Design review of the part built by this model. Coordinates are the model's own, in mm. A direction names the side the tool comes from. Coordinates: 2 decimals unless noted, no trailing zeros. Order: outer loops, then holes, each group sorted by start corner. A loop starts at its lowest first (then second) coordinate and runs counter-clockwise, first axis right, second up. Notation, with made-up numbers: (-8.75, 62.25) -> (1.25, 62.25) arc R19 ccw to (1.25, 82.25) -> close; hole circle Ø3 at (61, -38.75). An arc over 180 degrees is marked (long way). Use a Markdown table: item, result. Add a question column.
Q1. Machinability: for faces 4 (the face through (-3.4, 12.3, 7.5)), 5 (the face through (2.17, -9.76, -4.89)), 6 (the face through (-11.923, 3.755, -7.423)), which of the approach directions +Z, -Z, +X, -X, +Y, -Y give a long, thin tool a straight path to every point of the face, cutting with its end or side? Answer none if there is none.
Q2. Add section A-A (x = 0). State the section outline as (y, z) points.
Q3. Add section D-D (z = 3.75). State the section outline as (x, y) points.
Q4. Insertion check: pin 1 (2 mm diameter, centred on y = 10.5, z = 5, fed in from -X); pin 2 (4 mm diameter, centred on x = -6, z = 3.5, fed in from +Y); pin 3 (1 mm diameter, centred on x = 2.5, z = 0, fed in from -Y). Each pin has a flat end and moves straight along its axis. Give the tip position at first contact, or say it passes through.
Q5. The part is to be moulded in two halves that separate along Y. For faces 1 (the face through (-14.985, 0.66, 3.698)), 2 (the face through (0, 0, -15)), 3 (the face through (11.923, 3.755, 4.965)), say which applies: pulls with the +Y half, pulls with the -Y half, needs draft (parallel to the pull), parting line crosses it, or undercut.
Q6. Add section C-C (z = -3). State the section outline as (x, y) points.
Q7. Wall thickness on probe 1 along Y at (x, z) = (0, 5.65); probe 2 along Z at (x, y) = (-6, -5.5); probe 3 along X at (y, z) = (8, 0.5): over which ranges is each line inside the solid? List them lowest first.
from build123d import *

# Parameters (mm, degrees)
ESBO_O1_R                = 15
RESSALTO_EXTRUS_O1_DEPTH = 7.5
ESBO_O2_R                = 12.5
RESSALTO_EXTRUS_O2_DEPTH = 15
CASCA1_T                 = -2.5
FILETE2_R                = 2


with BuildPart() as part:
    # Esboço1 → Ressalto-extrusão1 (new body)
    with BuildSketch(Plane.XY):
        Circle(ESBO_O1_R)
    extrude(amount=RESSALTO_EXTRUS_O1_DEPTH)

    # Esboço2 → Ressalto-extrusão2 (add)
    with BuildSketch(Plane(origin=(0, 0, 0), x_dir=(-1, 0, 0), z_dir=(0, 0, -1))):
        Circle(ESBO_O2_R)
    extrude(amount=RESSALTO_EXTRUS_O2_DEPTH)

    # Casca1
    casca1_openings = [part.faces().sort_by_distance(p)[0] for p in [
        (0, 0, 7.5),
    ]]
    offset(amount=CASCA1_T, openings=casca1_openings, kind=Kind.INTERSECTION)

    # Filete2
    filete2_edges = [part.edges().sort_by_distance(p)[0] for p in [
        (12.5, 0, 0),
        (12.5, 0, -15),
    ]]
    fillet(filete2_edges, radius=FILETE2_R)


solid = part.part
Established:
| question | item | result |
|---|---|---|
| 1 | face 4 | +Z, +X, -X, +Y, -Y |
| 1 | face 5 | +Z |
| 1 | face 6 | -Z |
| 2 | outline | (-15, 0) -> (-14.5, 0) arc R2 cw to (-12.5, -2) -> (-12.5, -13) arc R2 ccw to (-10.5, -15) -> (10.5, -15) arc R2 ccw to (12.5, -13) -> (12.5, -2) arc R2 cw to (14.5, 0) -> (15, 0) -> (15, 7.5) -> (12.5, 7.5) -> (12.5, 2.5) -> (10, 2.5) -> (10, -12.5) -> (-10, -12.5) -> (-10, 2.5) -> (-12.5, 2.5) -> (-12.5, 7.5) -> (-15, 7.5) -> close |
| 3 | outline | circle Ø30 at (0, 0); hole circle Ø25 at (0, 0) |
| 4 | pin 1 | x = -11.61 |
| 4 | pin 2 | y = 14.46 |
| 4 | pin 3 | y = -14.87 |
| 5 | face 1 | parting line crosses it |
| 5 | face 2 | needs draft |
| 5 | face 3 | undercut |
| 6 | outline | circle Ø25 at (0, 0); hole circle Ø20 at (0, 0) |
| 7 | probe 1 | -15 to -12.5, 12.5 to 15 |
| 7 | probe 2 | -15 to -12.5 |
| 7 | probe 3 | -12.69 to -6, 6 to 12.69 |
